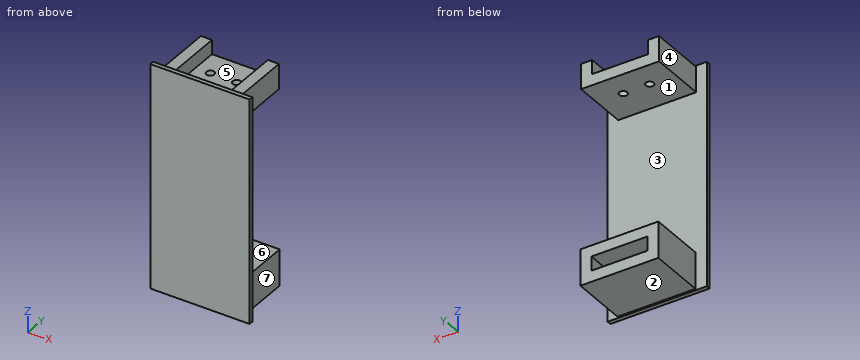
Solid Edge part; units mm, degrees
sketch "Sketch1" plane through (0, 0, 0) normal (0, 1, 0) x (-1, 0, 0)
  line L0 (-175, -395) -> (175, -395)
  line L1 (175, -395) -> (175, 395)
  line L2 (175, 395) -> (-175, 395)
  line L3 (-175, 395) -> (-175, -395)
  dimension "D1" = 175
  dimension "D2" = 175
extrude "Protrusion1" add sketch "Sketch1" against normal blind 15
sketch "Sketch2" plane through (0, 0, 0) normal (0, 1, 0) x (0, 0, -1)
  line L0 (-390, 137.5) -> (-301, 137.5)
  line L1 (-301, 137.5) -> (-301, -137.5)
  line L2 (-301, -137.5) -> (-390, -137.5)
  line L3 (-390, -137.5) -> (-390, 137.5)
  dimension "D1" = 390
  dimension "D2" = 301
extrude "ExtrudedProtrusion_4" add sketch "Sketch2" along normal blind 200
sketch "Sketch3" plane through (0, 0, 0) normal (0, 1, 0) x (0, 0, -1)
  line L0 (262, 135) -> (390, 135)
  line L1 (390, 135) -> (390, -140)
  line L2 (390, -140) -> (262, -140)
  line L3 (262, -140) -> (262, 135)
  dimension "D1" = 262
  dimension "D2" = 390
  dimension "D3" = 390
  dimension "D4" = 390
extrude "ExtrudedProtrusion_5" add sketch "Sketch3" along normal blind 200
sketch "Sketch4" plane through (0, 200, 355.5) normal (0, 1, 0) x (0, 0, -1)
  line L0 (-34.5, 98.5) -> (15.5, 98.5)
  line L1 (15.5, 98.5) -> (15.5, -98.5)
  line L2 (15.5, -98.5) -> (-34.5, -98.5)
  line L3 (-34.5, -98.5) -> (-34.5, 98.5)
extrude "ExtrudedCutout_1" cut sketch "Sketch4" against normal blind 200
sketch "Sketch5" plane through (2.5, 200, -355.5) normal (0, 1, 0) x (0, 0, -1)
  line L0 (-54.5, 98.5) -> (-4.5, 98.5)
  line L1 (-4.5, 98.5) -> (-4.5, -98.5)
  line L2 (-4.5, -98.5) -> (-54.5, -98.5)
  line L3 (-54.5, -98.5) -> (-54.5, 98.5)
  dimension "D1" = 54.5
extrude "ExtrudedCutout_2" cut sketch "Sketch5" against normal blind 200
sketch "Sketch6" plane through (0, 100, 340) normal (0, 0, 1) x (0, 1, 0)
  circle A0 centre (11.7858, -46.5) radius 14
  circle A1 centre (11.7858, 46.5) radius 14
  dimension "D1" = 11.7858
extrude "ExtrudedCutout_5" cut sketch "Sketch6" against normal blind 710
Geometry: final body of the model. Coordinates: model frame, mm. Face numbers are marked on the shaded views. A direction names the side the tool comes from. Round coordinates to 2 decimals unless told otherwise and drop trailing zeros. Order: outer loops, then holes, each group sorted by start corner. A loop starts at its lowest first (then second) coordinate and runs counter-clockwise, first axis right, second up. Notation, with made-up numbers: (88.25, -2.5) -> (100.25, -2.5) arc R18 ccw to (100.25, 6.5) -> close; hole circle Ø10 at (3.5, 19.25). An arc over 180 degrees is marked (long way). Use one line per item in the form item = value. Start each with the question number.
1. Cut plane A-A (y = 82). Return the cut outline in (x, z).
2. Cut plane B-B (x = 46.5). Return the cut outline in (y, z), then the cut area to 3 significant figures.
3. Cut plane D-D (z = -27.5). Return the cut outline in (x, y), then the cut area to 3 significant figures.
4. Draft query along X for the marked faces 4, 5, 6 and 7. Return one class per face: pulls with the +X half, pulls with the -X half, needs draft (parallel to the pull), parting line crosses it, or undercut.
5. Line query: probe 1 along Z at (x, y) = (-7, 93.5); probe 2 along X at (y, z) = (101, -340.5); probe 3 along Z at (x, y) = (115, 96). Output: solid intervals per line, ascending.
6. Reachability of the marked faces 1, 2 and 3 from +Z, -Z, +X, -X, +Y, -Y: full face, straight path, thin tool, end or side. Return the list, or none.
7. Cut plane C-C (x = -14). Return the cut outline in (y, z).
8. Pin query (flat end, axial travel): pin 1 Ø25 at (x, z) = (-32, -336) entering from +Y; pin 2 Ø25 at (x, y) = (46.5, 111.79) entering from -Z; pin 3 Ø2 at (x, y) = (131, 73) entering from +Z. Return the tip coordinate at first contact, or that it passes through.
Solution:
q1.outline = (-137.5, 301) -> (137.5, 301) -> (137.5, 390) -> (98.5, 390) -> (98.5, 340) -> (-98.5, 340) -> (-98.5, 390) -> (-137.5, 390) -> close; (-135, -390) -> (140, -390) -> (140, -262) -> (-135, -262) -> close; hole (-96, -351) -> (101, -351) -> (101, -301) -> (-96, -301) -> close
q2.outline = (-15, -395) -> (0, -395) -> (0, -390) -> (200, -390) -> (200, -351) -> (125.79, -351) -> (125.79, -370) -> (97.79, -370) -> (97.79, -351) -> (0, -351) -> (0, -301) -> (97.79, -301) -> (97.79, -262) -> (0, -262) -> (0, 301) -> (97.79, 301) -> (97.79, 340) -> (0, 340) -> (0, 395) -> (-15, 395) -> close; (125.79, -301) -> (200, -301) -> (200, -262) -> (125.79, -262) -> close; (125.79, 301) -> (200, 301) -> (200, 340) -> (125.79, 340) -> close
q2.area = 32,500 mm^2
q3.outline = (-175, -15) -> (175, -15) -> (175, 0) -> (-175, 0) -> close
q3.area = 5,250 mm^2
q4.face_4 = pulls with the -X half
q4.face_5 = undercut
q4.face_6 = needs draft
q4.face_7 = pulls with the +X half
q5.probe_1 = -390 to -351, -301 to -262, 301 to 340
q5.probe_2 = -135 to -96, 101 to 140
q5.probe_3 = -390 to -262, 301 to 390
q6.face_1 = +X, -X, +Y
q6.face_2 = -Z, +X, -X, +Y
q6.face_3 = +Y
q7.outline = (-15, -395) -> (0, -395) -> (0, -390) -> (200, -390) -> (200, -351) -> (0, -351) -> (0, -301) -> (200, -301) -> (200, -262) -> (0, -262) -> (0, 301) -> (200, 301) -> (200, 340) -> (0, 340) -> (0, 395) -> (-15, 395) -> close
q8.pin_1 = 0
q8.pin_2 = -390
q8.pin_3 = 390
